```python
from build123d import *
from build123d.topology import SkipClean

# Parameters (mm, degrees)
SKETCH1_R            = 40
SKETCH1_R_2          = 32
SKETCH1_R_3          = 5
BOSS_EXTRUDE1_DEPTH  = 4
SKETCH3_R            = 32
SKETCH3_R_2          = 5
CUT_EXTRUDE2_DEPTH   = 3
FILLET5_R            = 122
M5_CLEARANCE_HOLE1_D = 5.5


with BuildPart() as part:
    # Sketch1 → Boss-Extrude1 (new, symmetric)
    # profile 1 of 5: a face of its own
    with BuildSketch(Plane.XY):
        Circle(SKETCH1_R)
        Circle(SKETCH1_R_2, mode=Mode.SUBTRACT)
    # profile 2 of 5: a face of its own
    with BuildSketch(Plane.XY):
        with BuildLine():
            Line((-3, 31.859064644), (-3, 4))
            ThreePointArc((-3, 4), (0, 5), (3, 4))
            Line((3, 4), (3, 31.859064644))
            ThreePointArc((3, 31.859064644), (0, 32), (-3, 31.859064644))
        make_face()
    # profile 3 of 5: a face of its own
    with BuildSketch(Plane.XY):
        Circle(SKETCH1_R_3)
    # profile 4 of 5: a face of its own
    with BuildSketch(Plane.XY):
        with BuildLine():
            Line((29.090759323, -13.331456111), (4.964101615, 0.598076211))
            ThreePointArc((4.964101615, 0.598076211), (4.991017335, 0.299576304), (5, 0))
            ThreePointArc((5, 0), (4.172559651, -2.754949357), (1.964101615, -4.598076211))
            Line((1.964101615, -4.598076211), (26.090759323, -18.527608533))
            ThreePointArc((26.090759323, -18.527608533), (27.712812921, -16), (29.090759323, -13.331456111))
        make_face()
    # profile 5 of 5: a face of its own
    with BuildSketch(Plane.XY):
        with BuildLine():
            ThreePointArc((-1.964101615, -4.598076211), (-4.330127019, -2.5), (-4.964101615, 0.598076211))
            Line((-4.964101615, 0.598076211), (-29.090759323, -13.331456111))
            ThreePointArc((-29.090759323, -13.331456111), (-27.712812921, -16), (-26.090759323, -18.527608533))
            Line((-26.090759323, -18.527608533), (-1.964101615, -4.598076211))
        make_face()
    extrude(amount=BOSS_EXTRUDE1_DEPTH, both=True)

    # Sketch3 → Cut-Extrude2 (cut)
    with SkipClean():  # the faces are left unmerged after this step: merging them gives an invalid solid
        with BuildSketch(Plane.XY.offset(4)):
            with Locations(Location((0, 0, 0), (0, 0, 204.620621009))):
                Circle(SKETCH3_R)
            with Locations(Location((0, 0, 0), (0, 0, 173.130102354))):
                Circle(SKETCH3_R_2, mode=Mode.SUBTRACT)
        extrude(amount=-CUT_EXTRUDE2_DEPTH, mode=Mode.SUBTRACT)

    # Fillet5
    # the kernel refuses this fillet: 122 mm, written as the material it adds along each edge
    with BuildSketch(Plane(origin=(0, 0, 1), x_dir=(0.8644503363816339, 0.5027182271707281, 0), z_dir=(0.5027182271707281, -0.8644503363816339, 0))) as fillet5_piece_1_section:
        with BuildLine():
            CenterArc((31.888659319, 122), FILLET5_R, 257.267539737, 12.732460263)
            Line((31.888659319, 0), (5, 0))
            Line((5, 0), (5, 3))
        make_face()
    fillet5_piece_1 = revolve(axis=Axis((0, 0, 1), (0, 0, 1)), revolution_arc=359.64, mode=Mode.PRIVATE)
    fillet5_piece_1 = split(fillet5_piece_1, bisect_by=Plane(origin=(3, 0, 1), z_dir=(-1, 0, 0)), keep=Keep.TOP, mode=Mode.PRIVATE)
    fillet5_piece_1 = split(fillet5_piece_1, bisect_by=Plane(origin=(-1.5, 2.598076211, 1), z_dir=(0.5000000000000004, -0.8660254037844384, 0)), keep=Keep.TOP, mode=Mode.PRIVATE)
    fillet5_piece_1 = split(fillet5_piece_1, bisect_by=Plane(origin=(-1.5, -2.598076211, 1), z_dir=(0.49999999999999983, 0.8660254037844387, 0)), keep=Keep.TOP, mode=Mode.PRIVATE)
    add(fillet5_piece_1)
    with BuildSketch(Plane(origin=(0, 0, 1), x_dir=(0.8644503363816339, 0.5027182271707281, 0), z_dir=(0.5027182271707281, -0.8644503363816339, 0))) as fillet5_piece_2_section:
        with BuildLine():
            CenterArc((31.888659319, 122), FILLET5_R, 257.267539737, 12.732460263)
            Line((31.888659319, 0), (5, 0))
            Line((5, 0), (5, 3))
        make_face()
    fillet5_piece_2 = revolve(axis=Axis((0, 0, 1), (0, 0, 1)), revolution_arc=359.64, mode=Mode.PRIVATE)
    fillet5_piece_2 = split(fillet5_piece_2, bisect_by=Plane(origin=(3, 0, 1), z_dir=(-1, 0, 0)), keep=Keep.TOP, mode=Mode.PRIVATE)
    fillet5_piece_2 = split(fillet5_piece_2, bisect_by=Plane(origin=(-3, 0, 1), z_dir=(1, 0, 0)), keep=Keep.TOP, mode=Mode.PRIVATE)
    fillet5_piece_2 = split(fillet5_piece_2, bisect_by=Plane(origin=(1.5, -2.598076211, 1), z_dir=(-0.5000000000000003, 0.8660254037844385, 0)), keep=Keep.TOP, mode=Mode.PRIVATE)
    add(fillet5_piece_2)
    with BuildSketch(Plane(origin=(0, 0, 1), x_dir=(0.8644503363816339, 0.5027182271707281, 0), z_dir=(0.5027182271707281, -0.8644503363816339, 0))) as fillet5_piece_3_section:
        with BuildLine():
            CenterArc((31.888659319, 122), FILLET5_R, 257.267539737, 12.732460263)
            Line((31.888659319, 0), (5, 0))
            Line((5, 0), (5, 3))
        make_face()
    fillet5_piece_3 = revolve(axis=Axis((0, 0, 1), (0, 0, 1)), revolution_arc=359.64, mode=Mode.PRIVATE)
    fillet5_piece_3 = split(fillet5_piece_3, bisect_by=Plane(origin=(1.5, 2.598076211, 1), z_dir=(-0.49999999999999983, -0.8660254037844387, 0)), keep=Keep.TOP, mode=Mode.PRIVATE)
    fillet5_piece_3 = split(fillet5_piece_3, bisect_by=Plane(origin=(-1.5, 2.598076211, 1), z_dir=(0.5000000000000004, -0.8660254037844384, 0)), keep=Keep.TOP, mode=Mode.PRIVATE)
    fillet5_piece_3 = split(fillet5_piece_3, bisect_by=Plane(origin=(1.5, -2.598076211, 1), z_dir=(-0.5000000000000003, 0.8660254037844385, 0)), keep=Keep.TOP, mode=Mode.PRIVATE)
    add(fillet5_piece_3)
    with BuildSketch(Plane(origin=(0, 0, 1), x_dir=(0.8644503363816339, 0.5027182271707281, 0), z_dir=(0.5027182271707281, -0.8644503363816339, 0))) as fillet5_piece_4_section:
        with BuildLine():
            CenterArc((31.888659319, 122), FILLET5_R, 257.267539737, 12.732460263)
            Line((31.888659319, 0), (5, 0))
            Line((5, 0), (5, 3))
        make_face()
    fillet5_piece_4 = revolve(axis=Axis((0, 0, 1), (0, 0, 1)), revolution_arc=359.64, mode=Mode.PRIVATE)
    fillet5_piece_4 = split(fillet5_piece_4, bisect_by=Plane(origin=(1.5, 2.598076211, 1), z_dir=(-0.49999999999999983, -0.8660254037844387, 0)), keep=Keep.TOP, mode=Mode.PRIVATE)
    fillet5_piece_4 = split(fillet5_piece_4, bisect_by=Plane(origin=(1.5, -2.598076211, 1), z_dir=(0.5000000000000003, -0.8660254037844385, 0)), keep=Keep.TOP, mode=Mode.PRIVATE)
    fillet5_piece_4 = split(fillet5_piece_4, bisect_by=Plane(origin=(-1.5, -2.598076211, 1), z_dir=(0.49999999999999983, 0.8660254037844387, 0)), keep=Keep.TOP, mode=Mode.PRIVATE)
    add(fillet5_piece_4)
    with BuildSketch(Plane(origin=(0, 0, 1), x_dir=(-0.8675919238668259, 0.4972768380299447, 0), z_dir=(0.4972768380299447, 0.8675919238668259, 0))) as fillet5_piece_5_section:
        with BuildLine():
            CenterArc((31.888659319, 122), FILLET5_R, 257.267539737, 12.732460263)
            Line((31.888659319, 0), (5, 0))
            Line((5, 0), (5, 3))
        make_face()
    fillet5_piece_5 = revolve(axis=Axis((0, 0, 1), (0, 0, 1)), revolution_arc=359.64, mode=Mode.PRIVATE)
    fillet5_piece_5 = split(fillet5_piece_5, bisect_by=Plane(origin=(1.5, 2.598076211, 1), z_dir=(-0.49999999999999983, -0.8660254037844387, 0)), keep=Keep.TOP, mode=Mode.PRIVATE)
    fillet5_piece_5 = split(fillet5_piece_5, bisect_by=Plane(origin=(-1.5, 2.598076211, 1), z_dir=(0.5000000000000004, -0.8660254037844384, 0)), keep=Keep.TOP, mode=Mode.PRIVATE)
    fillet5_piece_5 = split(fillet5_piece_5, bisect_by=Plane(origin=(-1.5, -2.598076211, 1), z_dir=(0.49999999999999983, 0.8660254037844387, 0)), keep=Keep.TOP, mode=Mode.PRIVATE)
    add(fillet5_piece_5)
    with BuildSketch(Plane(origin=(0, 0, 1), x_dir=(-0.8675919238668259, 0.4972768380299447, 0), z_dir=(0.4972768380299447, 0.8675919238668259, 0))) as fillet5_piece_6_section:
        with BuildLine():
            CenterArc((31.888659319, 122), FILLET5_R, 257.267539737, 12.732460263)
            Line((31.888659319, 0), (5, 0))
            Line((5, 0), (5, 3))
        make_face()
    fillet5_piece_6 = revolve(axis=Axis((0, 0, 1), (0, 0, 1)), revolution_arc=359.64, mode=Mode.PRIVATE)
    fillet5_piece_6 = split(fillet5_piece_6, bisect_by=Plane(origin=(3, 0, 1), z_dir=(-1, 0, 0)), keep=Keep.TOP, mode=Mode.PRIVATE)
    fillet5_piece_6 = split(fillet5_piece_6, bisect_by=Plane(origin=(-1.5, 2.598076211, 1), z_dir=(0.5000000000000004, -0.8660254037844384, 0)), keep=Keep.TOP, mode=Mode.PRIVATE)
    fillet5_piece_6 = split(fillet5_piece_6, bisect_by=Plane(origin=(1.5, -2.598076211, 1), z_dir=(-0.5000000000000003, 0.8660254037844385, 0)), keep=Keep.TOP, mode=Mode.PRIVATE)
    add(fillet5_piece_6)
    with BuildSketch(Plane(origin=(0, 0, 1), x_dir=(-0.8675919238668259, 0.4972768380299447, 0), z_dir=(0.4972768380299447, 0.8675919238668259, 0))) as fillet5_piece_7_section:
        with BuildLine():
            CenterArc((31.888659319, 122), FILLET5_R, 257.267539737, 12.732460263)
            Line((31.888659319, 0), (5, 0))
            Line((5, 0), (5, 3))
        make_face()
    fillet5_piece_7 = revolve(axis=Axis((0, 0, 1), (0, 0, 1)), revolution_arc=359.64, mode=Mode.PRIVATE)
    fillet5_piece_7 = split(fillet5_piece_7, bisect_by=Plane(origin=(3, 0, 1), z_dir=(-1, 0, 0)), keep=Keep.TOP, mode=Mode.PRIVATE)
    fillet5_piece_7 = split(fillet5_piece_7, bisect_by=Plane(origin=(-3, 0, 1), z_dir=(1, 0, 0)), keep=Keep.TOP, mode=Mode.PRIVATE)
    fillet5_piece_7 = split(fillet5_piece_7, bisect_by=Plane(origin=(-1.5, -2.598076211, 1), z_dir=(0.49999999999999983, 0.8660254037844387, 0)), keep=Keep.TOP, mode=Mode.PRIVATE)
    add(fillet5_piece_7)
    with BuildSketch(Plane(origin=(0, 0, 1), x_dir=(0.0031415874858787157, -0.9999950652018581, 0), z_dir=(-0.9999950652018581, -0.0031415874858787157, 0))) as fillet5_piece_8_section:
        with BuildLine():
            CenterArc((31.888659319, 122), FILLET5_R, 257.267539737, 12.732460263)
            Line((31.888659319, 0), (5, 0))
            Line((5, 0), (5, 3))
        make_face()
    fillet5_piece_8 = revolve(axis=Axis((0, 0, 1), (0, 0, 1)), revolution_arc=359.64, mode=Mode.PRIVATE)
    fillet5_piece_8 = split(fillet5_piece_8, bisect_by=Plane(origin=(1.5, 2.598076211, 1), z_dir=(-0.49999999999999983, -0.8660254037844387, 0)), keep=Keep.TOP, mode=Mode.PRIVATE)
    fillet5_piece_8 = split(fillet5_piece_8, bisect_by=Plane(origin=(-1.5, 2.598076211, 1), z_dir=(0.5000000000000004, -0.8660254037844384, 0)), keep=Keep.TOP, mode=Mode.PRIVATE)
    fillet5_piece_8 = split(fillet5_piece_8, bisect_by=Plane(origin=(-1.5, -2.598076211, 1), z_dir=(0.49999999999999983, 0.8660254037844387, 0)), keep=Keep.TOP, mode=Mode.PRIVATE)
    add(fillet5_piece_8)
    with BuildSketch(Plane(origin=(0, 0, 1), x_dir=(0.0031415874858787157, -0.9999950652018581, 0), z_dir=(-0.9999950652018581, -0.0031415874858787157, 0))) as fillet5_piece_9_section:
        with BuildLine():
            CenterArc((31.888659319, 122), FILLET5_R, 257.267539737, 12.732460263)
            Line((31.888659319, 0), (5, 0))
            Line((5, 0), (5, 3))
        make_face()
    fillet5_piece_9 = revolve(axis=Axis((0, 0, 1), (0, 0, 1)), revolution_arc=359.64, mode=Mode.PRIVATE)
    fillet5_piece_9 = split(fillet5_piece_9, bisect_by=Plane(origin=(3, 0, 1), z_dir=(-1, 0, 0)), keep=Keep.TOP, mode=Mode.PRIVATE)
    fillet5_piece_9 = split(fillet5_piece_9, bisect_by=Plane(origin=(-3, 0, 1), z_dir=(1, 0, 0)), keep=Keep.TOP, mode=Mode.PRIVATE)
    fillet5_piece_9 = split(fillet5_piece_9, bisect_by=Plane(origin=(1.5, -2.598076211, 1), z_dir=(-0.5000000000000003, 0.8660254037844385, 0)), keep=Keep.TOP, mode=Mode.PRIVATE)
    add(fillet5_piece_9)
    with BuildSketch(Plane(origin=(0, 0, 1), x_dir=(0.0031415874858787157, -0.9999950652018581, 0), z_dir=(-0.9999950652018581, -0.0031415874858787157, 0))) as fillet5_piece_10_section:
        with BuildLine():
            CenterArc((31.888659319, 122), FILLET5_R, 257.267539737, 12.732460263)
            Line((31.888659319, 0), (5, 0))
            Line((5, 0), (5, 3))
        make_face()
    fillet5_piece_10 = revolve(axis=Axis((0, 0, 1), (0, 0, 1)), revolution_arc=359.64, mode=Mode.PRIVATE)
    fillet5_piece_10 = split(fillet5_piece_10, bisect_by=Plane(origin=(-1.5, 2.598076211, 1), z_dir=(0.5000000000000004, -0.8660254037844384, 0)), keep=Keep.TOP, mode=Mode.PRIVATE)
    fillet5_piece_10 = split(fillet5_piece_10, bisect_by=Plane(origin=(1.5, -2.598076211, 1), z_dir=(-0.5000000000000003, 0.8660254037844385, 0)), keep=Keep.TOP, mode=Mode.PRIVATE)
    fillet5_piece_10 = split(fillet5_piece_10, bisect_by=Plane(origin=(-1.5, -2.598076211, 1), z_dir=(-0.49999999999999983, -0.8660254037844387, 0)), keep=Keep.TOP, mode=Mode.PRIVATE)
    add(fillet5_piece_10)

    # M5 Clearance Hole1 (through all)
    with Locations(Plane.XY.offset(4)):
        with Locations((0, 0)):
            Hole(M5_CLEARANCE_HOLE1_D / 2)


solid = part.part
```
The listing builds one solid part. Answer for the finished solid, in the listing's coordinates (mm). A direction names the side the tool comes from. Give positions to 0.01 mm unless a question says otherwise; leave off trailing zeros. Order: outer loops, then holes, each group sorted by start corner. A loop starts at its lowest first (then second) coordinate and runs counter-clockwise, first axis right, second up. Notation, with made-up numbers: (-40, 63) -> (16, 63) arc R21 cw to (16, 76) -> close; hole circle Ø1 at (-27.75, -6). An arc over 180 degrees is marked (long way). One line per item, written item: value.
1) Find the intervals of material crossed by line 1 (X direction, y = 14.5, z = -1.25); line 2 (Y direction, x = -5, z = 0.5); line 3 (Y direction, x = 4, z = -1), in increasing order.
Reported:
line 1: x = -37.28 to -28.53, -3 to 3, 28.53 to 37.28
line 2: y = -39.69 to -31.61, -6.35 to 0.58, 31.61 to 39.69
line 3: y = -39.8 to -31.75, -5.77 to 3, 31.75 to 39.8
2) A tool of negligible diameter and unlimited length cuts with its end or side. For faces 4 (the cylindrical face through (0, -5, 0)), 5 (the flat face through (2.2, -2.2, 4)), from which of +Z, -Z, +X, -X, +Y, -Y can it reach the whole face along a straight path? Write none if from no direction.
Reported:
face 4: +Z, -Z
face 5: +Z, +X, -X, +Y, -Y
3) Determine the mould class of faces 1 (the cylindrical face through (-8.67, -39.05, 0.06)), 2 (the flat face through (-1, 9, -4)), 3 (the cylindrical face through (4.34, 2.48, 0.06)) for opening direction X: pulls with the +X half, pulls with the -X half, needs draft (parallel to the pull), parting line crosses it, or undercut.
Reported:
face 1: parting line crosses it
face 2: needs draft
face 3: undercut
4) Flat-ended cylindrical pins translate along their axes: P1, Ø3, axis at y = 2.5, z = -1, coming from the +X side; P2, Ø2.5, axis at y = 17.5, z = 0, coming from the -X side; P3, Ø1.5, axis at y = 6.5, z = -2, coming from the -X side. Find the tip coordinate at first contact, or state that the pin passes through.
Reported:
P1: stops at x = 39.99
P2: stops at x = -36.55
P3: stops at x = -39.58
5) Find section B-B, the plane x = 0. Count the separate pieces of the cut face and the enclosed holes in it, plus the area to 3 significant figures.
Reported:
separate pieces: 3
enclosed holes: 0
area: 326 mm^2
6) Find section A-A, the plane z = -0.25. Determine the outline of the cut face in (x, y), plus the area to 3 significant figures.
Reported:
outline: circle Ø80 at (0, 0); hole (-29.09, -13.33) -> (-4.96, 0.6) arc R5 cw to (-3, 4) -> (-3, 31.86) arc R32 ccw to start; hole (-26.09, -18.53) arc R32 ccw to (26.09, -18.53) -> (1.96, -4.6) arc R5 cw to (-1.96, -4.6) -> close; hole circle Ø5.5 at (0, 0); hole (3, 4) arc R5 cw to (4.96, 0.6) -> (29.09, -13.33) arc R32 ccw to (3, 31.86) -> close
area: 2,360 mm^2
